Can you work these out from the model? Positions are in its coordinate system, mm. A direction names the side the tool comes from. Give positions to 0.01 mm unless a question says otherwise; leave off trailing zeros. Loops run counter-clockwise (first coordinate to the right, second up) from the corner with the lowest first, then second, coordinate; pieces in that order, holes last. Notation, with made-up numbers: (5.5, -17.75) - (15.5, -17.75) arc R28 ccw to (15.5, 15.25) - close; hole circle Ø10 at (-35, -32.5). An arc over 180 degrees is marked (long way). Answer as a JSON object with one key per item and string values.
```python
from build123d import *

# Parameters (mm, degrees)
BOSS_EXTRUDE1_DEPTH = 30
SKETCH2_R           = 2.5
BOSS_EXTRUDE2_DEPTH = 3
FILLET1_R           = 10


with BuildPart() as part:
    # Sketch1 → Boss-Extrude1 (new body)
    with BuildSketch(Plane.XY):
        with BuildLine():
            Line((-20, 20), (0, 20))
            Line((0, 20), (0, 12.5))
            ThreePointArc((0, 12.5), (-12.5, 0), (0, -12.5))
            Line((0, -12.5), (0, -20))
            Line((0, -20), (-20, -20))
            Line((-20, -20), (-20, 20))
        make_face()
    extrude(amount=BOSS_EXTRUDE1_DEPTH)

    # Sketch2 → Boss-Extrude2 (add)
    with BuildSketch(Plane(origin=(0, 0, 0), x_dir=(-1, 0, 0), z_dir=(0, 0, -1))):
        with BuildLine():
            Line((0, -12.5), (0, -3))
            ThreePointArc((0, -3), (3, 0), (0, 3))
            Line((0, 3), (0, 12.5))
            ThreePointArc((0, 12.5), (12.5, 0), (0, -12.5))
        make_face()
        with Locations((8.5, 0)):
            Circle(SKETCH2_R, mode=Mode.SUBTRACT)
    extrude(amount=-BOSS_EXTRUDE2_DEPTH)

    # Fillet1
    fillet1_edges = [part.edges().sort_by_distance(p)[0] for p in [
        (-20, -20, 15),
        (-20, 20, 15),
    ]]
    fillet(fillet1_edges, radius=FILLET1_R)


solid = part.part
```
1) Imagine slicing it at B-B on z = 2. Write out the boundary of the cut face in (x, y), and give its area (3 significant figures).
Check sheet entries:
{"outline": "(-20, -10) arc R10 ccw to (-10, -20) - (0, -20) - (0, -3) arc R3 cw to (0, 3) - (0, 20) - (-10, 20) arc R10 ccw to (-20, 10) - close; hole circle Ø5 at (-8.5, 0)", "area": "723 mm2"}
2) If we mould it in two halves opening along X, with no side actions, what happens to faces 1 (the flat face through (-14, 0, 30)), 2 (the cylindrical face through (-10.885, 0.751, 1.479)), 3 (the flat face through (0, -15, 15)), 4 (the cylindrical face through (-16.99, 17.15, 15.21))? For each: released by +X, released by -X, zero draft, split by the parting line, or undercut.
Check sheet entries:
{"face 1": "zero draft", "face 2": "undercut", "face 3": "released by +X", "face 4": "released by -X"}
3) I need wall thicknesses on L1, parallel to Y at x = -8.5, z = 2.45; L2, parallel to Y at x = -2.5, z = 6.75; L3, parallel to Z at x = -5.75, y = 4.5. Which ranges of each line are inside material? Lowest first, please.
Check sheet entries:
{"L1": "-20 to -2.5, 2.5 to 20", "L2": "-20 to -12.25, 12.25 to 20", "L3": "0 to 3"}
4) Imagine slicing it at C-C on x = -9.5. Write out the boundary of the cut face in (y, z), and give its area (3 significant figures).
Check sheet entries:
{"outline": "(-20, 0) - (-2.29, 0) - (-2.29, 3) - (-8.12, 3) - (-8.12, 30) - (-20, 30) - close; (2.29, 0) - (20, 0) - (20, 30) - (8.12, 30) - (8.12, 3) - (2.29, 3) - close", "area": "748 mm2"}
5) I'm going to push a flat-ended pin straight in: P1, Ø4, axis at x = -4, y = 2, coming from the +Z side. Where does the tip first touch, or does it pass through?
Check sheet entries:
{"P1": "z = 3"}
6) Imagine slicing it at A-A on y = 0. Write out the boundary of the cut face in (x, z), and give its area (4 significant figures).
Check sheet entries:
{"outline": "(-20, 0) - (-11, 0) - (-11, 3) - (-12.5, 3) - (-12.5, 30) - (-20, 30) - close; (-6, 0) - (-3, 0) - (-3, 3) - (-6, 3) - close", "area": "238.5 mm2"}
7) Imagine slicing it at D-D on y = 16. Write out the boundary of the cut face in (x, z), and give its area (3 significant figures).
Check sheet entries:
{"outline": "(-18, 0) - (0, 0) - (0, 30) - (-18, 30) - close", "area": "540 mm2"}
8) Which directions (+Z, -Z, +X, -X, +Y, -Y) give clear straight access to the entire face, cutting with the end or side of a thin tool? Please do faces 5 (the flat face through (-5, 0, 3)), 6 (the flat face through (-5, -20, 15)).
Check sheet entries:
{"face 5": "+Z, +X", "face 6": "+Z, -Z, +X, -X, -Y"}
